Read the model definition and answer for the solid it produces. Units are mm, in the model's axes. Face numbers are marked on the shaded views. A direction names the side the tool comes from. Coordinates: 2 decimals unless noted, no trailing zeros. Order: outer loops, then holes, each group sorted by start corner. A loop starts at its lowest first (then second) coordinate and runs counter-clockwise, first axis right, second up. Notation, with made-up numbers: (30, 81) - (76, 81) arc R11 cw to (76, 101) - close; hole circle Ø8 at (41, -16.5). An arc over 180 degrees is marked (long way). Use one line per item in the form item = value.
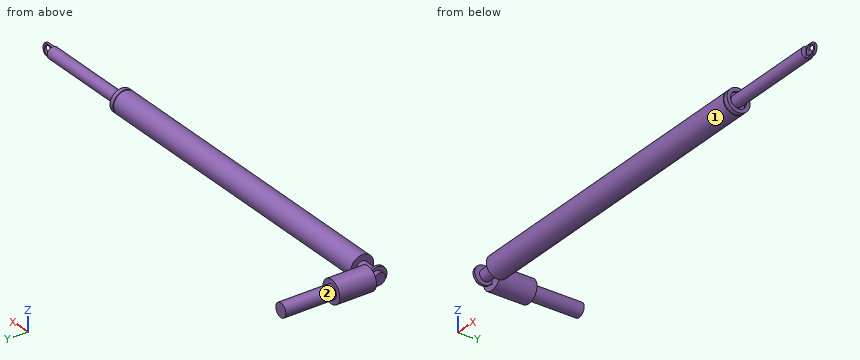
```python
from build123d import *

# Parameters (mm, degrees)
SKETCH_2_R          = 2.5
EXTRUDE_2_DEPTH     = 7.5
SKETCH_10_R         = 3
EXTRUDE_3_DEPTH     = 15
SKETCH_11_R         = 5
EXTRUDE_4_DEPTH     = 16
SKETCH_12_W         = 1
SKETCH_12_H         = 5
EXTRUDE_6_DEPTH     = 0.4
EXTRUDE_7_DEPTH     = 1
SKETCH_14_R         = 2.5
EXTRUDE_10_DEPTH    = 2
EXTRUDE_START       = 2
SKETCH_21_R         = 3
EXTRUDE_14_DEPTH    = 2
SKETCH_25_R         = 5
EXTRUDE_16_DEPTH    = 144
SKETCH_26_R         = 3.5
CUT_EXTRUDE_3_DEPTH = 1
SKETCH_27_R         = 2.5
EXTRUDE_17_DEPTH    = 42
EXTRUDE_18_DEPTH    = 0.5
SKETCH_19_R         = 2.103210471
CUT_EXTRUDE_4_DEPTH = 0.5
EXTRUDE_START_2     = 3
SKETCH_31_R         = 3
EXTRUDE_19_DEPTH    = 3
SKETCH_32_R         = 3
EXTRUDE_20_DEPTH    = 2
SKETCH_33_OUTSIDE_W = 53.63
SKETCH_33_OUTSIDE_H = 89.578
SKETCH_33_OUTSIDE_R = 4.8
CUT_EXTRUDE_6_DEPTH = 0.25


with BuildPart() as part:
    # Sketch 2 → Extrude 2 (new body)
    with BuildSketch(Plane(origin=(0, 0, 0), x_dir=(0, 0, -1), z_dir=(1, 0, 0))):
        with Locations((0, 12.052457573)):
            Circle(SKETCH_2_R)
    extrude(amount=EXTRUDE_2_DEPTH)



with BuildPart() as body_2:
    # Sketch 10 → Extrude 3 (new body)
    with BuildSketch(Plane(origin=(0, 45.94754243, 0), x_dir=(1, 0, 0), z_dir=(0, 1, 0))):
        with Locations(Location((0, 0, 0), (0, 0, 270))):
            Circle(SKETCH_10_R)
    extrude(amount=-EXTRUDE_3_DEPTH)

    # Sketch 11 → Extrude 4 (add)
    with BuildSketch(Plane(origin=(0, 30.94754243, 0), x_dir=(1, 0, 0), z_dir=(0, 1, 0))):
        with Locations(Location((0, 0, 0), (0, 0, 270))):
            Circle(SKETCH_11_R)
    extrude(amount=-EXTRUDE_4_DEPTH)


with BuildPart() as part_1:
    add(part.part)

    add(body_2.part)  # Extrude 6 merges body 2
    # Sketch 12 → Extrude 6 (add)
    with BuildSketch(Plane.XZ.offset(-14.94754243)):
        with Locations((-0.5, 0.028858947)):
            Rectangle(SKETCH_12_W, SKETCH_12_H)
    extrude(amount=EXTRUDE_6_DEPTH)

    # Sketch 13 → Extrude 7 (add)
    with BuildSketch(Plane(origin=(0, 0, 0), x_dir=(0, 0, -1), z_dir=(1, 0, 0))):
        with BuildLine():
            Line((-2.528858947, 14.54754243), (2.471141053, 14.54754243))
            ThreePointArc((2.471141053, 14.54754243), (-0.028858947, 7.425043431), (-2.528858947, 14.54754243))
        make_face()
    extrude(amount=-EXTRUDE_7_DEPTH)

    # Sketch 14 → Extrude 10 (add)
    with BuildSketch(Plane.ZY.offset(1)):
        with Locations(Location((0.028858947, 12.04754243, 0), (0, 0, 180))):
            Circle(SKETCH_14_R)
    extrude(amount=EXTRUDE_10_DEPTH)

    # Sketch 21 → Extrude 14 (add)
    with BuildSketch(Plane(origin=(0, 45.94754243, 0), x_dir=(1, 0, 0), z_dir=(0, 1, 0)).offset(EXTRUDE_START)):
        with Locations(Location((0, 0, 0), (0, 0, 270))):
            Circle(SKETCH_21_R)
    extrude(amount=-EXTRUDE_14_DEPTH)

    # Sketch 25 → Extrude 16 (add)
    with BuildSketch(Plane(origin=(7.5, 0, 0), x_dir=(0, 0, -1), z_dir=(1, 0, 0))):
        with Locations((0, 12)):
            Circle(SKETCH_25_R)
    extrude(amount=EXTRUDE_16_DEPTH)

    # Sketch 26 → Cut-Extrude 3 (cut)
    with BuildSketch(Plane(origin=(151.5, 0, 0), x_dir=(0, 0, -1), z_dir=(1, 0, 0))):
        with Locations((0, 12)):
            Circle(SKETCH_26_R)
    extrude(amount=-CUT_EXTRUDE_3_DEPTH, mode=Mode.SUBTRACT)

    # Sketch 27 → Extrude 17 (add)
    with BuildSketch(Plane(origin=(150.5, 0, 0), x_dir=(0, 0, -1), z_dir=(1, 0, 0))):
        with Locations((0, 12)):
            Circle(SKETCH_27_R)
    extrude(amount=EXTRUDE_17_DEPTH)

    # Sketch 30 → Extrude 18 (add, symmetric)
    with BuildSketch(Plane(origin=(0, 12, 0), x_dir=(1, 0, 0), z_dir=(0, 1, 0))):
        with BuildLine():
            Line((192.5, 2.5), (196.5, 2.5))
            ThreePointArc((196.5, 2.5), (197.767182761, 0), (196.5, -2.5))
            Line((196.5, -2.5), (192.5, -2.5))
            Line((192.5, -2.5), (192.5, 2.5))
        make_face()
    extrude(amount=EXTRUDE_18_DEPTH, both=True)

    # Sketch 19 → Cut-Extrude 4 (cut, symmetric)
    with BuildSketch(Plane(origin=(0, 12, 0), x_dir=(1, 0, 0), z_dir=(0, 1, 0))):
        with Locations(Location((194.882176, 0, 0), (0, 0, 270))):
            Circle(SKETCH_19_R)
    extrude(amount=CUT_EXTRUDE_4_DEPTH, both=True, mode=Mode.SUBTRACT)

    # Sketch 31 → Extrude 19 (add)
    with BuildSketch(Plane(origin=(0, 47.94754243, 0), x_dir=(1, 0, 0), z_dir=(0, 1, 0)).offset(EXTRUDE_START_2)):
        with Locations(Location((0, 0, 0), (0, 0, 270))):
            Circle(SKETCH_31_R)
    extrude(amount=-EXTRUDE_19_DEPTH)

    # Sketch 32 → Extrude 20 (add)
    with BuildSketch(Plane(origin=(0, 50.94754243, 0), x_dir=(1, 0, 0), z_dir=(0, 1, 0)).offset(EXTRUDE_START)):
        with Locations(Location((0, 0, 0), (0, 0, 270))):
            Circle(SKETCH_32_R)
    extrude(amount=-EXTRUDE_20_DEPTH)

    # Sketch 33 outside → Cut-Extrude 6 (cut, symmetric)
    with BuildSketch(Plane(origin=(149.5, 0, 0), x_dir=(0, 0, -1), z_dir=(1, 0, 0))):
        with Locations((0, 29.974)):
            Rectangle(SKETCH_33_OUTSIDE_W, SKETCH_33_OUTSIDE_H)
        with Locations((0, 12)):
            Circle(SKETCH_33_OUTSIDE_R, mode=Mode.SUBTRACT)
    extrude(amount=CUT_EXTRUDE_6_DEPTH, both=True, mode=Mode.SUBTRACT)


solid = part_1.part
```
(1) Section B-B, the plane x = 90.5 is taken. Write down the section's boundary in (y, z).
Answer list:
outline = circle Ø10 at (12, 0)
(2) Given pin 1 Ø4 at (y, z) = (12.5, 0) entering from -X; pin 2 Ø4 at (x, z) = (195.5, 1) entering from +Y; pin 3 Ø0.8 at (x, y) = (193.5, 12) entering from +Z, each flat-ended and moving along its own axis, determine where each tip first touches the part or whether it passes through.
Answer list:
pin_1 = -3
pin_2 = 12.5
pin_3 = 2.5
(3) Which of the six approach directions +Z, -Z, +X, -X, +Y, -Y give full straight-line access (tool end or side, diameter ignored) to the marked faces 1 and 2?
Answer list:
face_1 = +X
face_2 = +Y
(4) Section A-A, the plane y = 44 is taken. Write down the section's boundary in (x, z), then the cut area to 3 significant figures.
Answer list:
outline = circle Ø6 at (0, 0)
area = 28.3 mm2
(5) Straight lines are drawn through the part: L1, parallel to Y at x = 150.8, z = 0; L2, parallel to X at y = 11.8, z = 0; L3, parallel to X at y = 25.5, z = 4. For each, find the intervals that lie inside material, in ascending order.
Answer list:
L1 = 7 to 8.5, 9.5 to 14.5, 15.5 to 17
L2 = -3 to 192.78, 196.99 to 197.77
L3 = -3 to 3
